Build history of the part. All positions in model axes, mm. A direction names the side the tool comes from. Give positions to 0.01 mm unless a question says otherwise; leave off trailing zeros. Loops run counter-clockwise (first coordinate to the right, second up) from the corner with the lowest first, then second, coordinate; pieces in that order, holes last. Notation, with made-up numbers: (31, -39.75) - (75, -39.75) arc R13 cw to (75, -26.75) - close; hole circle Ø5 at (54.25, 83). An arc over 180 degrees is marked (long way). Return JSON: item names as keys, results as strings. Group by question number.
1) Slice it at A-A (z = 61). List the corners of the cut face in (x, y), and give its area (3 significant figures).
2) Drop a flat-ended pin along its axis: pin 1 (2 mm diameter, centred on x = -51, y = -72.5, fed in from +Z). Give the stop position or say it passes through.
3) Mould opens along Y. For faces 3 (the face through (-272.5, 236, 46)), 4 (the face through (-3, 2, 80)) say: released by +Y, released by -Y, zero draft, split by the parting line, or undercut.
4) Drill centre lines: probe 1 along Y at (x, z) = (-182, 19); probe 2 along X at (y, z) = (-186, 18); probe 3 along Z at (x, y) = (-100, 233). Where is each one in solid material? Low to high. Write a range as from..to.
5) Slice it at C-C (y = 66.5). List the corners of the cut face in (x, z), and give its area (3 significant figures).
6) Slice it at B-B (x = -447). List the corners of the cut face in (y, z).
7) 3-axis set-ups, long thin cutter, end or side, ignore diameter. For faces 1 (the face through (-4, 454, 46)), 2 (the face through (-595, -6, 39)): which of +Z, -Z, +X, -X, +Y, -Y reach the whole face in a straight line?
```python
from build123d import *

# Parameters (mm, degrees)
F0_W     = 1190
F0_H     = 920
F1_DEPTH = 80
F2_W     = 1178
F2_H     = 908
F3_DEPTH = 68
F4_W     = 50
F4_H     = 80
F5_DEPTH = 908
F6_W     = 50
F6_H     = 80
F7_DEPTH = 1178


with BuildPart() as f1:
    # F0 (on Top) → F1 (new body)
    with BuildSketch(Plane.XY):
        Rectangle(F0_W, F0_H)
    extrude(amount=F1_DEPTH)

    # F2 (on face) → F3 (cut)
    with BuildSketch(Plane.XY.offset(80)):
        Rectangle(F2_W, F2_H)
    extrude(amount=-F3_DEPTH, mode=Mode.SUBTRACT)

    # F4 (on face) → F5 (join)
    with BuildSketch(Plane(origin=(0, -454, 0), x_dir=(-1, 0, 0), z_dir=(0, 1, 0))):
        with Locations((-297.5, 40)):
            Rectangle(F4_W, F4_H)
        with Locations((297.5, 40)):
            Rectangle(F4_W, F4_H)
    extrude(amount=F5_DEPTH)

    # F6 (on face) → F7 (join)
    with BuildSketch(Plane(origin=(589, 0, 0), x_dir=(0, -1, 0), z_dir=(-1, 0, 0))):
        with Locations((0, 40)):
            Rectangle(F6_W, F6_H)
    extrude(amount=F7_DEPTH)


solid = f1.part
```
Results:
{
 "1": {"outline": "(-595, -460) - (595, -460) - (595, 460) - (-595, 460) - close; hole (-589, -454) - (-322.5, -454) - (-322.5, -25) - (-589, -25) - close; hole (-589, 25) - (-322.5, 25) - (-322.5, 454) - (-589, 454) - close; hole (-272.5, -454) - (272.5, -454) - (272.5, -25) - (-272.5, -25) - close; hole (-272.5, 25) - (272.5, 25) - (272.5, 454) - (-272.5, 454) - close; hole (322.5, -454) - (589, -454) - (589, -25) - (322.5, -25) - close; hole (322.5, 25) - (589, 25) - (589, 454) - (322.5, 454) - close", "area": "170,000 mm2"},
 "2": {"pin 1": "z = 12"},
 "3": {"face 3": "undercut", "face 4": "zero draft"},
 "4": {"probe 1": "-460..-454, -25..25, 454..460", "probe 2": "-595..-589, -322.5..-272.5, 272.5..322.5, 589..595", "probe 3": "0..12"},
 "5": {"outline": "(-595, 0) - (595, 0) - (595, 80) - (589, 80) - (589, 12) - (322.5, 12) - (322.5, 80) - (272.5, 80) - (272.5, 12) - (-272.5, 12) - (-272.5, 80) - (-322.5, 80) - (-322.5, 12) - (-589, 12) - (-589, 80) - (-595, 80) - close", "area": "21,900 mm2"},
 "6": {"outline": "(-460, 0) - (460, 0) - (460, 80) - (454, 80) - (454, 12) - (25, 12) - (25, 80) - (-25, 80) - (-25, 12) - (-454, 12) - (-454, 80) - (-460, 80) - close"},
 "7": {"face 1": "+Z", "face 2": "+Z, -Z, -X, +Y, -Y"}
}
